Source: three-view drawing plus pictorial views. Frame: mm from the lowest corner of the part. A direction names the side the tool comes from. Round coordinates to 2 decimals unless told otherwise and drop trailing zeros. Write each loop counter-clockwise with the first axis right and the second up, starting at its lowest first coordinate (ties: lowest second). Pieces come first, ordered by that corner, then holes. Notation, with made-up numbers: M 7,63 L 59,63 A18 ccw 59,83 Z; hole C 27.25,23 d1. An arc over 180 degrees is marked long. Put each result on its own line as item: value. Start each with the question number.
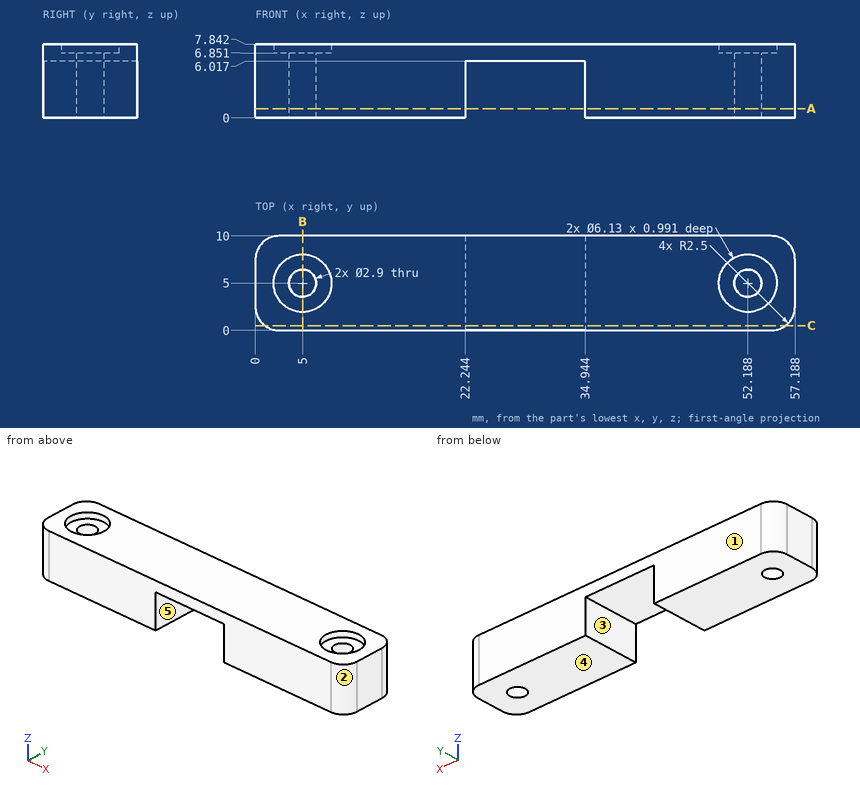
(1) Ray query, line 1 along X through (y, z) = (5, 3.25); line 2 along X through (y, z) = (5.75, 2.5); line 3 along X through (y, z) = (3.25, 0.5). Return the intervals inside material, ascending.
(2) Contact query for flat-ended pins moving along their axis: P1, Ø5, axis at x = 52.188, y = 5, coming from the +Z side; P2, Ø2, axis at x = 33, y = 5, coming from the -Z side; P3, Ø3, axis at y = 7, z = 3, coming from the -X side. Output: stop coordinate, or through.
(3) Pull-direction query (X, two-part tool) for the marked faces 1, 2 and 3; classes: +X half, -X half, draft (parallel to the pull), parting line (faces both ways), or undercut.
(4) Section query B-B (x = 5). Return loops of the section in (y, z) (3 decimals).
(5) Section query C-C (y = 0.5). Return loops of the section in (x, z), and give its area (3 significant figures).
(6) Section query A-A (z = 1). Return loops of the section in (x, y).
(7) Access query for the marked faces 4 and 5. Directions: +Z, -Z, +X, -X, +Y, -Y. A direction counts if a zero-diameter tool reaches every point of the face in a straight line with its end or side. Return the directions, or none.
Entries:
1. line 1: 0 to 3.55, 6.45 to 22.24, 34.94 to 50.74, 53.64 to 57.19
1. line 2: 0 to 3.76, 6.24 to 22.24, 34.94 to 50.95, 53.43 to 57.19
1. line 3: 0 to 22.24, 34.94 to 57.19
2. P1: z = 6.85
2. P2: z = 6.02
2. P3: x = 0
3. face 1: draft
3. face 2: +X half
3. face 3: undercut
4. outline: M 0,0 L 3.55,0 L 3.55,6.851 L 1.935,6.851 L 1.935,7.842 L 0,7.842 Z; M 6.45,0 L 10,0 L 10,7.842 L 8.065,7.842 L 8.065,6.851 L 6.45,6.851 Z
5. outline: M 1,0 L 22.24,0 L 22.24,6.02 L 34.94,6.02 L 34.94,0 L 56.19,0 L 56.19,7.84 L 1,7.84 Z
5. area: 356 mm2
6. outline: M 0,2.5 A2.5 ccw 2.5,0 L 22.24,0 L 22.24,10 L 2.5,10 A2.5 ccw 0,7.5 Z; M 34.94,0 L 54.69,0 A2.5 ccw 57.19,2.5 L 57.19,7.5 A2.5 ccw 54.69,10 L 34.94,10 Z; hole C 5,5 d2.9; hole C 52.19,5 d2.9
7. face 4: -Z, +X, -X, +Y, -Y
7. face 5: -Z, +Y, -Y
